Source: CAD feature listing. Evaluate the final solid. Frame: model axes, mm. Round coordinates to 2 decimals unless told otherwise and drop trailing zeros. Write each loop counter-clockwise with the first axis right and the second up, starting at its lowest first coordinate (ties: lowest second). Pieces come first, ordered by that corner, then holes. Notation, with made-up numbers: M -11,-29.5 L 44,-29.5 A13 ccw 44,-25.5 Z; hole C 70,21 d4. An arc over 180 degrees is marked long. Put each result on its own line as item: value. Start each with the question number.
```python
from build123d import *

# Parameters (mm, degrees)
ESQUISSE1_W             = 155
ESQUISSE1_H             = 30
BOSS_EXTRU_1_DEPTH      = 5
ESQUISSE2_R             = 1.5
ESQUISSE2_R_2           = 0.5
BOSS_EXTRU_2_DEPTH      = 4
CONG_1_R                = 1
ESQUISSE4_W             = 5
ESQUISSE4_H             = 30
ENL_V_MAT_EXTRU_2_DEPTH = 17


with BuildPart() as part:
    # Esquisse1 → Boss.-Extru.1 (new body)
    with BuildSketch(Plane.XY):
        Rectangle(ESQUISSE1_W, ESQUISSE1_H)
    extrude(amount=BOSS_EXTRU_1_DEPTH)

    # Esquisse2 → Boss.-Extru.2 (add)
    # profile 1 of 2: a face of its own
    with BuildSketch(Plane(origin=(0, 15, 0), x_dir=(1, 0, 0), z_dir=(0, 1, 0))):
        with Locations(Location((-38.75, -2.5, 0), (0, 0, 90))):
            Circle(ESQUISSE2_R)
        with Locations(Location((-38.75, -2.5, 0), (0, 0, 270))):
            Circle(ESQUISSE2_R_2, mode=Mode.SUBTRACT)
    # profile 2 of 2: a face of its own
    with BuildSketch(Plane(origin=(0, 15, 0), x_dir=(1, 0, 0), z_dir=(0, 1, 0))):
        with Locations(Location((38.75, -2.5, 0), (0, 0, 90))):
            Circle(ESQUISSE2_R)
        with Locations(Location((38.75, -2.5, 0), (0, 0, 270))):
            Circle(ESQUISSE2_R_2, mode=Mode.SUBTRACT)
    extrude(amount=BOSS_EXTRU_2_DEPTH)

    # Congé1
    cong_1_edges = [part.edges().sort_by_distance(p)[0] for p in [
        (-38.75, 19, 4),
        (38.75, 19, 4),
    ]]
    fillet(cong_1_edges, radius=CONG_1_R - 0.0001)  # a hair under: the kernel refuses the full size

    # Esquisse4 → Enlèv. mat.-Extru.2 (cut)
    with BuildSketch(Plane(origin=(77.5, 0, 0), x_dir=(0, 0, -1), z_dir=(1, 0, 0))):
        with Locations((-2.5, 0)):
            Rectangle(ESQUISSE4_W, ESQUISSE4_H)
    extrude(amount=-ENL_V_MAT_EXTRU_2_DEPTH, mode=Mode.SUBTRACT)


solid = part.part
```
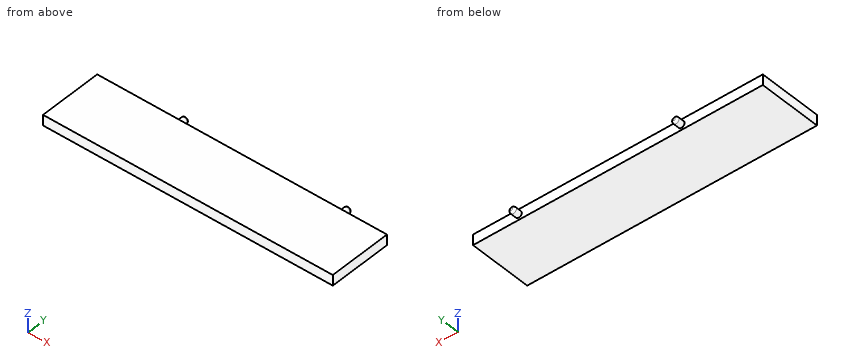
(1) Contact query for a flat-ended pin moving along its axis: P1, Ø1.5, axis at x = -18, z = 1.5, coming from the +Y side. Output: stop coordinate, or through.
(2) Section query A-A (x = -9). Return loops of the section in (y, z), and give its area (3 significant figures).
(3) Ray query, line 1 along X through (y, z) = (16.95, 2.5); line 2 along Z through (x, y) = (38.75, 17.65); line 3 along Y through (x, z) = (-42.5, 0.85). Return the intervals inside material, ascending.
Entries:
1. P1: y = 15
2. outline: M -15,0 L 15,0 L 15,5 L -15,5 Z
2. area: 150 mm2
3. line 1: -40.25 to -39.25, -38.25 to -37.25, 37.25 to 38.25, 39.25 to 40.25
3. line 2: 1 to 2, 3 to 4
3. line 3: -15 to 15
